from build123d import *

# Parameters (mm, degrees)
SKETCH6_R           = 45
BOSS_EXTRUDE7_DEPTH = 100
SKETCH8_R           = 40
BOSS_EXTRUDE8_DEPTH = 40


with BuildPart() as part:
    # Sketch6 → Boss-Extrude7 (new body)
    with BuildSketch(Plane(origin=(0, 0, 0), x_dir=(1, 0, 0), z_dir=(0, 1, 0))):
        with Locations(Location((0, 0, 0), (0, 0, 270))):
            Circle(SKETCH6_R)
    extrude(amount=BOSS_EXTRUDE7_DEPTH)


with BuildPart() as body_2:
    # Sketch7 → Revolve2 (revolve)
    with BuildSketch(Plane.XY, mode=Mode.PRIVATE) as revolve2_sk:
        with BuildLine():
            Line((0, 100), (0, 125.083403494))
            Line((0, 125.083403494), (-88.216224583, 125.083403494))
            Line((-88.216224583, 125.083403494), (-88.216224583, 0))
            Line((-88.216224583, 0), (-45, 0))
            add(Edge.make_bspline(
                [(-45, 0), (-45.199870538, 9.069967987), (-45.686940304, 37.078388642), (-29.510811545, 88.131965608), (0, 100)],
                knots=[0, 0, 0, 0, 0.165319882, 1, 1, 1, 1], degree=3))
        make_face()
    revolve(revolve2_sk.sketch.rotate(Axis((0, 100, 0), (0, 1, 0)), 180), axis=Axis((0, 100, 0), (0, 1, 0)))


with BuildPart() as part_1:
    add(part.part)

    # Intersect1: read off the stored shape, not the designer's step
    # Intersect1: cut body 2
    add(body_2.part, mode=Mode.SUBTRACT)

    # Sketch8 → Boss-Extrude8 (add)
    with BuildSketch(Plane.XZ):
        with Locations(Location((0, 0, 0), (0, 0, 270))):
            Circle(SKETCH8_R)
    extrude(amount=BOSS_EXTRUDE8_DEPTH)


solid = part_1.part
The listing builds one solid part. Answer for the finished solid, in the listing's coordinates (mm). A direction names the side the tool comes from. Give positions to 0.01 mm unless a question says otherwise; leave off trailing zeros.
1) Find the intervals of material crossed by L1, parallel to Z at x = -5, y = 50; L2, parallel to X at y = -31.5, z = 1.5; L3, parallel to X at y = 15, z = -33, in increasing order.
2) A tool of negligible diameter and unlimited length cuts with its end or side. For faces 1 (the face through (1, -40, 1)), 2 (the face through (-39.05, -19.72, 8.67)), from which of +Z, -Z, +X, -X, +Y, -Y can it reach the whole face along a straight path? Write none if from no direction.
3) Given P1, Ø8, axis at y = 20, z = 9, coming from the +X side; P2, Ø3, axis at y = 1, z = 18, coming from the +X side; P3, Ø1, axis at x = -17.5, z = -22, coming from the +Y side, each flat-ended and moving along its own axis, determine where each tip first touches the part or whether it passes through.
Response:
1. L1: z = -38.38 to 38.38
1. L2: x = -39.97 to 39.97
1. L3: x = -30.59 to 30.59
2. face 1: +Z, -Z, +X, -X, -Y
2. face 2: -Y
3. P1: stops at x = 44.63
3. P2: stops at x = 41.87
3. P3: stops at y = 74.65
